Drawing for the job (mm, zero at the part's lowest x, y, z). A direction names the side the tool comes from. Give positions to 0.01 mm unless a question says otherwise; leave off trailing zeros. Write each loop counter-clockwise with the first axis right and the second up, starting at its lowest first coordinate (ties: lowest second). Pieces come first, ordered by that corner, then holes. Notation, with made-up numbers: M -29,76.5 L 14,76.5 A29 ccw 14,105.5 Z; hole C 88.25,42 d6. An arc over 180 degrees is marked long. Use CSV: the item, a comma, the result in double quotes. Start each with the question number.
1. Band-saw the part on B-B, the plane y = 56. List the corners of the cut face in (x, z).
2. Drop flat-ended pins along their axis: pin 1 Ø1.5 at (y, z) = (48.5, 25) entering from +X; pin 2 Ø10 at (x, z) = (25, 35) entering from -Y; pin 3 Ø17 at (y, z) = (11, 11) entering from +X. Give the stop position or say it passes through.
3. Band-saw the part on A-A, the plane z = 20. List the corners of the cut face in (x, y), then the cut area to 3 significant figures.
4. Band-saw the part on C-C, the plane x = 7. List the corners of the cut face in (y, z).
5. Mould opens along X. For the marked faces 1, 2 and 3 say: pulls with the +X half, pulls with the -X half, needs draft (parallel to the pull), parting line crosses it, or undercut.
6. 3-axis set-ups, long thin cutter, end or side, ignore diameter. For the marked faces 4, 5, 6 and 7: which of +Z, -Z, +X, -X, +Y, -Y reach the whole face in a straight line?
7. Drill centre lines: line 1 along Z through (x, y) = (7, 56); line 2 along Y through (x, z) = (93, 34.5); line 3 along X through (y, z) = (5.5, 19). Where is each one in solid material? Low to high. Write a range as from..to.
8. Band-saw the part on D-D, the plane z = 33. List the corners of the cut face in (x, y).
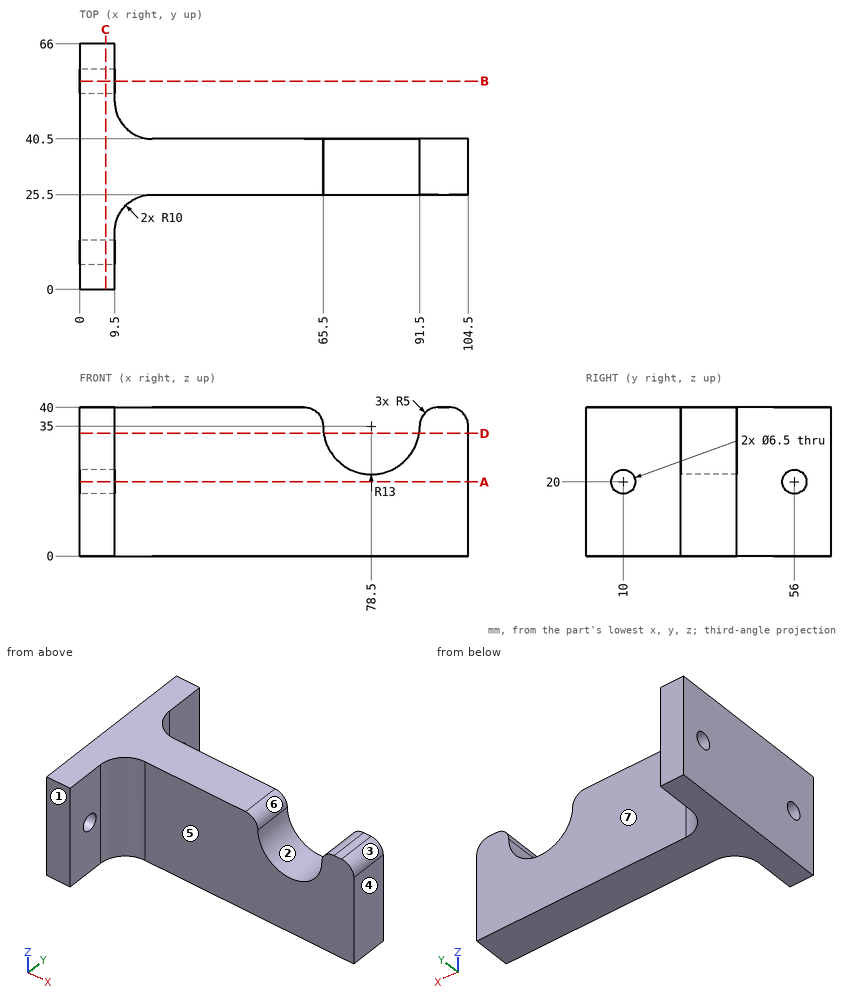
Output:
1,outline,"M 0,0 L 9.5,0 L 9.5,16.75 L 0,16.75 Z; M 0,23.25 L 9.5,23.25 L 9.5,40 L 0,40 Z"
2,pin 1,"stops at x = 9.89"
2,pin 2,"stops at y = 25.5"
2,pin 3,"stops at x = 10.33"
3,outline,"M 0,0 L 9.5,0 L 9.5,6.75 L 0,6.75 Z; M 0,13.25 L 9.5,13.25 L 9.5,15.5 A10 cw 19.5,25.5 L 104.5,25.5 L 104.5,40.5 L 19.5,40.5 A10 cw 9.5,50.5 L 9.5,52.75 L 0,52.75 Z; M 0,59.25 L 9.5,59.25 L 9.5,66 L 0,66 Z"
3,area,"1,970 mm²"
4,outline,"M 0,0 L 66,0 L 66,40 L 0,40 Z; hole C 10,20 d6.5; hole C 56,20 d6.5"
5,face 1,"needs draft"
5,face 2,"undercut"
5,face 3,"pulls with the +X half"
6,face 4,"+Z, -Z, +X, +Y, -Y"
6,face 5,"+Z, -Z, +X, -Y"
6,face 6,"+Z, +Y, -Y"
6,face 7,"+Z, -Z, +X, +Y"
7,line 1,"z = 0..16.75, 23.25..40"
7,line 2,"y = 25.5..40.5"
7,line 3,"x = 0..9.5"
8,outline,"M 0,0 L 9.5,0 L 9.5,15.5 A10 cw 19.5,25.5 L 65.65,25.5 L 65.65,40.5 L 19.5,40.5 A10 cw 9.5,50.5 L 9.5,66 L 0,66 Z; M 91.35,25.5 L 104.5,25.5 L 104.5,40.5 L 91.35,40.5 Z"
